```python
from build123d import *

# Parameters (mm, degrees)
SKETCH1_W           = 9.85
SKETCH1_H           = 4.75
SKETCH1_H_2         = 0.05
SKETCH1_W_2         = 0.05
SKETCH1_H_3         = 10.95
SKETCH1_W_3         = 0.25
BOSS_EXTRUDE1_DEPTH = 0.3
SKETCH2_W           = 1
SKETCH2_H           = 15.75
BOSS_EXTRUDE2_DEPTH = 1.6
SKETCH1_3_W         = 0.25
SKETCH1_3_H         = 10.95
CUT_EXTRUDE2_DEPTH  = 10


with BuildPart() as part:
    # Sketch1 → Boss-Extrude1 (new body)
    with BuildSketch(Plane(origin=(0, 0, 0), x_dir=(1, 0, 0), z_dir=(0, 1, 0))):
        with Locations((-5.275, 13.375)):
            Rectangle(SKETCH1_W, SKETCH1_H)
        with Locations((5.275, 13.375)):
            Rectangle(SKETCH1_W, SKETCH1_H)
        with Locations((-5.275, 10.975)):
            Rectangle(SKETCH1_W, SKETCH1_H_2)
        with Locations((5.275, 10.975)):
            Rectangle(SKETCH1_W, SKETCH1_H_2)
        Polygon((-0.35, 11), (-0.35, 10.95), (0.35, 10.95), (0.35, 11), (0.3, 11), (-0.3, 11), align=None)
        Polygon((-10.2, 10.95), (-10.2, 0), (10.2, 0), (10.2, 10.95), (0.35, 10.95), (-0.35, 10.95), align=None)
        with Locations((-10.225, 5.475)):
            Rectangle(SKETCH1_W_2, SKETCH1_H_3)
        with Locations((-10.375, 5.475)):
            Rectangle(SKETCH1_W_3, SKETCH1_H_3)
        with Locations((10.375, 5.475)):
            Rectangle(SKETCH1_W_3, SKETCH1_H_3)
        with Locations((10.225, 5.475)):
            Rectangle(SKETCH1_W_2, SKETCH1_H_3)
    extrude(amount=BOSS_EXTRUDE1_DEPTH)

    # Sketch2 → Boss-Extrude2 (add)
    with BuildSketch(Plane(origin=(0, 0.3, 0), x_dir=(1, 0, 0), z_dir=(0, 1, 0))):
        with Locations((-0.85, 7.875)):
            Rectangle(SKETCH2_W, SKETCH2_H)
        with Locations((0.85, 7.875)):
            Rectangle(SKETCH2_W, SKETCH2_H)
    extrude(amount=BOSS_EXTRUDE2_DEPTH)

    # Sketch1_3 → Cut-Extrude2 (cut)
    with BuildSketch(Plane(origin=(0, 0, 0), x_dir=(1, 0, 0), z_dir=(0, 1, 0))):
        with Locations((-10.375, 5.475)):
            Rectangle(SKETCH1_3_W, SKETCH1_3_H)
        with Locations((10.375, 5.475)):
            Rectangle(SKETCH1_3_W, SKETCH1_3_H)
    extrude(amount=CUT_EXTRUDE2_DEPTH, mode=Mode.SUBTRACT)


solid = part.part
```
The listing builds one solid part. Answer for the finished solid, in the listing's coordinates (mm). A direction names the side the tool comes from. Give positions to 0.01 mm unless a question says otherwise; leave off trailing zeros. Order: outer loops, then holes, each group sorted by start corner. A loop starts at its lowest first (then second) coordinate and runs counter-clockwise, first axis right, second up. Notation, with made-up numbers: M 71.5,79.5 L 91.5,79.5 A37 ccw 91.5,117.5 Z; hole C 31,15 d9. An arc over 180 degrees is marked long. Put each result on its own line as item: value. Start each with the question number.
Item 1: Flat-ended cylindrical pins translate along their axes: P1, Ø4.5, axis at x = -5, z = -11.5, coming from the +Y side; P2, Ø0.5, axis at y = 1, z = -7, coming from the +X side; P3, Ø0.6, axis at y = 1.5, z = -7, coming from the -X side. Find the tip coordinate at first contact, or state that the pin passes through.
Item 2: The part is cut by section C-C, the plane x = -6. Determine the outline of the cut face in (y, z), and give its area (4 significant figures).
Item 3: Find the intervals of material crossed by line 1 along X through (y, z) = (1.75, -3.25); line 2 along Y through (x, z) = (-5, -1), in increasing order.
Item 4: The part is cut by section B-B, the plane z = -6.25. Determine the outline of the cut face in (x, y), and give its area (3 significant figures).
Item 5: The part is cut by section A-A, the plane y = 1.15. Determine the outline of the cut face in (x, z).
Item 6: Which of the six approach directions +Z, -Z, +X, -X, +Y, -Y give full straight-line access (tool end or side, diameter ignored) to faces 1 (the face through (-0.8, 0.5, 0)), 2 (the face through (6, 0.3, -8)), 3 (the face through (-6, 0.3, -8))?
Answer key:
1. P1: stops at y = 0.3
1. P2: stops at x = 1.35
1. P3: stops at x = -1.35
2. outline: M 0,-15.75 L 0.3,-15.75 L 0.3,0 L 0,0 Z
2. area: 4.725 mm²
3. line 1: x = -1.35 to -0.35, 0.35 to 1.35
3. line 2: y = 0 to 0.3
4. outline: M -10.25,0 L 10.25,0 L 10.25,0.3 L 1.35,0.3 L 1.35,1.9 L 0.35,1.9 L 0.35,0.3 L -0.35,0.3 L -0.35,1.9 L -1.35,1.9 L -1.35,0.3 L -10.25,0.3 Z
4. area: 9.35 mm²
5. outline: M -1.35,-15.75 L -0.35,-15.75 L -0.35,0 L -1.35,0 Z; M 0.35,-15.75 L 1.35,-15.75 L 1.35,0 L 0.35,0 Z
6. face 1: +Z, +X, -X, +Y, -Y
6. face 2: +Z, -Z, +X, +Y
6. face 3: +Z, -Z, -X, +Y
